Could you check a few things on this model? Use its own coordinates, in mm. Face numbers are marked on the shaded views. Round coordinates to 2 decimals unless told otherwise and drop trailing zeros. Write each loop counter-clockwise with the first axis right and the second up, starting at its lowest first coordinate (ties: lowest second). Pieces come first, ordered by that corner, then holes. Notation, with made-up numbers: (12, 53.25) - (62, 53.25) arc R12 ccw to (62, 62.25) - close; hole circle Ø5 at (-37.75, 14). An arc over 180 degrees is marked (long way). Put each result on its own line as item: value.
from build123d import *

# Parameters (mm, degrees)
BOSS_EXTRUDE1_DEPTH = 8
SKETCH7_OUTSIDE_W   = 26.674
SKETCH7_OUTSIDE_H   = 27.518
SKETCH7_OUTSIDE_R   = 7.5
CUT_EXTRUDE4_DEPTH  = 1
CUT_EXTRUDE4_TAPER  = 60
SKETCH8_OUTSIDE_W   = 26.674
SKETCH8_OUTSIDE_H   = 27.518
SKETCH8_OUTSIDE_R   = 7.5
CUT_EXTRUDE5_DEPTH  = 1
CUT_EXTRUDE5_TAPER  = 60
SKETCH9_R           = 5
CUT_EXTRUDE6_DEPTH  = 10


with BuildPart() as part:
    # Sketch1 → Boss-Extrude1 (new body)
    with BuildSketch(Plane(origin=(0, 0, 0), x_dir=(1, 0, 0), z_dir=(0, 1, 0))):
        Polygon((6.673205692, -5.519812116), (8.116900362, 3.019259596), (1.44369467, 8.539071712), (-6.673205692, 5.519812116), (-8.116900362, -3.019259596), (-1.44369467, -8.539071712), align=None)
    extrude(amount=BOSS_EXTRUDE1_DEPTH)

    # Sketch7 outside → Cut-Extrude4 (cut)
    with BuildSketch(Plane(origin=(0, 8, 0), x_dir=(1, 0, 0), z_dir=(0, 1, 0))):
        Rectangle(SKETCH7_OUTSIDE_W, SKETCH7_OUTSIDE_H)
        Circle(SKETCH7_OUTSIDE_R, mode=Mode.SUBTRACT)
    extrude(amount=-CUT_EXTRUDE4_DEPTH, taper=CUT_EXTRUDE4_TAPER, mode=Mode.SUBTRACT)

    # Sketch8 outside → Cut-Extrude5 (cut)
    with BuildSketch(Plane.XZ):
        Rectangle(SKETCH8_OUTSIDE_W, SKETCH8_OUTSIDE_H)
        Circle(SKETCH8_OUTSIDE_R, mode=Mode.SUBTRACT)
    extrude(amount=-CUT_EXTRUDE5_DEPTH, taper=CUT_EXTRUDE5_TAPER, mode=Mode.SUBTRACT)

    # Sketch9 → Cut-Extrude6 (cut)
    with BuildSketch(Plane(origin=(0, 8, 0), x_dir=(1, 0, 0), z_dir=(0, 1, 0))):
        Circle(SKETCH9_R)
    extrude(amount=-CUT_EXTRUDE6_DEPTH, mode=Mode.SUBTRACT)


solid = part.part
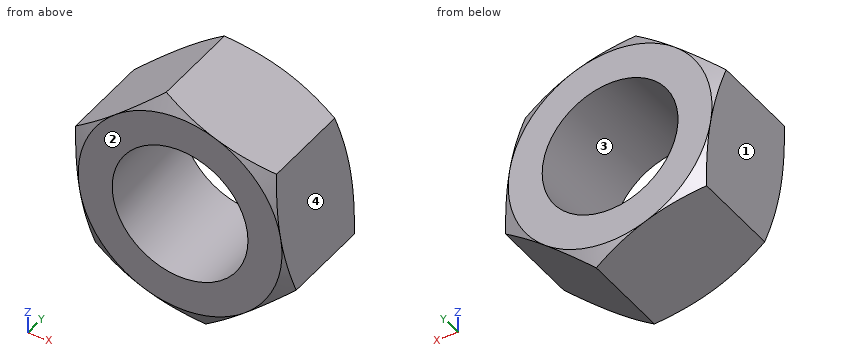
(1) I'm going to push flat-ended pins straight in: pin 1 (1.5 mm diameter, centred on y = 1.5, z = -5.5, fed in from -X); pin 2 (2 mm diameter, centred on y = 1, z = -1.5, fed in from +X); pin 3 (3 mm diameter, centred on x = 6.5, y = 5.5, fed in from -Z); pin 4 (8 mm diameter, centred on x = 0, z = 0, fed in from +Y). Where does each tip first touch, or does it pass through?
Values found:
pin 1: stops at x = -6.8
pin 2: stops at x = 8.03
pin 3: stops at z = -5.6
pin 4: passes through
(2) Imagine slicing it at B-B, the plane x = 0. List the corners of the cut face in (y, z) for me, then the cut area to 3 significant figures.
Values found:
outline: (0, -7.5) - (0.29, -8) - (7.71, -8) - (8, -7.5) - (8, -5) - (0, -5) - close; (0, 5) - (8, 5) - (8, 7.5) - (7.71, 8) - (0.29, 8) - (0, 7.5) - close
area: 47.7 mm^2
(3) Please list where these lines run through material, in increasing order: probe 1 along X at (y, z) = (2, 0); probe 2 along X at (y, z) = (6.75, 3); probe 3 along Z at (x, y) = (-0.75, 0.5). Write a range as from..to.
Values found:
probe 1: x = -7.61..-5, 5..7.61
probe 2: x = -8.11..-4, 4..7.1
probe 3: z = -7.72..-4.94, 4.94..8.28
(4) Imagine slicing it at A-A, the plane y = 5.75. List the corners of the cut face in (x, z) for me, then the cut area to 3 significant figures.
Values found:
outline: (-8.12, 3.02) - (-6.67, -5.52) - (1.44, -8.54) - (8.12, -3.02) - (6.67, 5.52) - (-1.44, 8.54) - close; hole circle Ø10 at (0, 0)
area: 116 mm^2
(5) If we mould it in two halves opening along X, with no side actions, what happens to the marked faces 1, 2, 3 and 4? For each: pulls with the +X half, pulls with the -X half, needs draft (parallel to the pull), parting line crosses it, or undercut.
Values found:
face 1: pulls with the -X half
face 2: needs draft
face 3: undercut
face 4: pulls with the +X half
